```python
from build123d import *

# Parameters (mm, degrees)
F0_W     = 660
F0_H     = 638
F1_DEPTH = 185
F2_R     = 80
F3_R     = 62.5
F4_DEPTH = 185.001
F5_R     = 35
F6_DEPTH = 185.001


with BuildPart() as f1:
    # F0 (on Right) → F1 (new body)
    with BuildSketch(Plane.YZ):
        Rectangle(F0_W, F0_H)
    extrude(amount=F1_DEPTH)

    # F2
    f2_edges = [f1.edges().sort_by_distance(p)[0] for p in [
        (92.5, 330, 319),
        (92.5, -330, 319),
        (92.5, 330, -319),
        (92.5, -330, -319),
    ]]
    fillet(f2_edges, radius=F2_R)

    # F3 (on face) → F4 (cut, through all)
    with BuildSketch(Plane.YZ.offset(185)):
        Circle(F3_R)
    extrude(amount=-F4_DEPTH, mode=Mode.SUBTRACT)

    # F5 (on face) → F6 (cut, through all)
    with BuildSketch(Plane.YZ.offset(185)):
        with Locations((-265, 240)):
            Circle(F5_R)
        with Locations((265, 240)):
            Circle(F5_R)
        with Locations((265, -240)):
            Circle(F5_R)
        with Locations((-265, -240)):
            Circle(F5_R)
    extrude(amount=-F6_DEPTH, mode=Mode.SUBTRACT)


solid = f1.part
```
Here's how the part is built. I have some questions about the finished solid (model axes, mm). Coordinates: 2 decimals unless noted, no trailing zeros. Write each loop counter-clockwise with the first axis right and the second up, starting at its lowest first coordinate (ties: lowest second). Pieces come first, ordered by that corner, then holes. Notation, with made-up numbers: (38, 39.25) -> (81, 39.25) arc R36 ccw to (81, 77.25) -> close; hole circle Ø2 at (22.5, -26). An arc over 180 degrees is marked (long way). Use a Markdown table: item, result. Add a question column.
(1) If we section it at A-A, the plane z = -24: Write out the boundary of the cut face in (x, y).
(2) If we section it at B-B, the plane y = 0: Write out the boundary of the cut face in (x, z).
(3) Please list where these lines run through material, in increasing order: line 1 (Z direction, x = 112, y = 0); line 2 (Z direction, x = 111.5, y = 265); line 3 (Y direction, x = 34.5, z = 3.5).
(4) We'd pull the mould along Y, two halves only. Please class faces 1 (the cylindrical face through (93.8, -62.44, 2.75)), 2 (the cylindrical face through (93.8, -246.18, -210.49)), 3 (the flat face through (0, -5, -66)), 4 (the cylindrical face through (93.8, 307.19, 294.94)): +Y half, -Y half, draft (parallel to the pull), parting line (faces both ways), or undercut.
(5) If we section it at C-C, the plane x = 173.5: Write out the boundary of the cut face in (y, z), and give its area (3 significant figures).
(6) If we section it at D-D, the plane y = 282: Write out the boundary of the cut face in (x, z), and give its area (3 significant figures).
Outcome:
| question | item | result |
|---|---|---|
| 1 | outline | (0, -330) -> (185, -330) -> (185, -57.71) -> (0, -57.71) -> close; (0, 57.71) -> (185, 57.71) -> (185, 330) -> (0, 330) -> close |
| 2 | outline | (0, -319) -> (185, -319) -> (185, -62.5) -> (0, -62.5) -> close; (0, 62.5) -> (185, 62.5) -> (185, 319) -> (0, 319) -> close |
| 3 | line 1 | z = -319 to -62.5, 62.5 to 319 |
| 3 | line 2 | z = -317.58 to -275, -205 to 205, 275 to 317.58 |
| 3 | line 3 | y = -330 to -62.4, 62.4 to 330 |
| 4 | face 1 | undercut |
| 4 | face 2 | undercut |
| 4 | face 3 | draft |
| 4 | face 4 | +Y half |
| 5 | outline | (-330, -239) arc R80 ccw to (-250, -319) -> (250, -319) arc R80 ccw to (330, -239) -> (330, 239) arc R80 ccw to (250, 319) -> (-250, 319) arc R80 ccw to (-330, 239) -> close; hole circle Ø70 at (-265, -240); hole circle Ø70 at (-265, 240); hole circle Ø125 at (0, 0); hole circle Ø70 at (265, -240); hole circle Ø70 at (265, 240) |
| 5 | area | 388,000 mm^2 |
| 6 | outline | (0, -312.32) -> (185, -312.32) -> (185, -270.59) -> (0, -270.59) -> close; (0, -209.41) -> (185, -209.41) -> (185, 209.41) -> (0, 209.41) -> close; (0, 270.59) -> (185, 270.59) -> (185, 312.32) -> (0, 312.32) -> close |
| 6 | area | 92,900 mm^2 |
